from build123d import *

# Parameters (mm, degrees)
SKETCH2_R           = 1.55
CUT_EXTRUDE5_DEPTH  = 14.87
CUT_EXTRUDE10_DEPTH = 3.88
SKETCH5_R           = 3.26
CUT_EXTRUDE11_DEPTH = 2.18


with BuildPart() as part:
    # Sketch1 → Revolve1 (revolve)
    with BuildSketch(Plane.XY):
        with BuildLine():
            Line((0, 0.5), (5.525741394, 0.5))
            ThreePointArc((5.525741394, 0.5), (7.89, 0), (5.525741394, -0.5))
            Line((5.525741394, -0.5), (4.86, -0.5))
            ThreePointArc((4.86, -0.5), (4.294314575, -0.734314575), (4.06, -1.3))
            Line((4.06, -1.3), (4.06, -5.55))
            ThreePointArc((4.06, -5.55), (3.825685425, -6.115685425), (3.26, -6.35))
            Line((3.26, -6.35), (0, -6.35))
            Line((0, -6.35), (0, 0))
            Line((0, 0), (0, 0.5))
        make_face()
    revolve(axis=Axis((0, 0, 0), (0, 1, 0)))

    # Sketch2 → Cut-Extrude5 (cut)
    with BuildSketch(Plane(origin=(0, 0.5, 0), x_dir=(1, 0, 0), z_dir=(0, 1, 0))):
        with Locations(Location((0, 0, 0), (0, 0, 180))):
            Circle(SKETCH2_R)
    extrude(amount=-CUT_EXTRUDE5_DEPTH, mode=Mode.SUBTRACT)

    # Sketch3 → Cut-Extrude10 (cut)
    with BuildSketch(Plane(origin=(0, 0.5, 0), x_dir=(1, 0, 0), z_dir=(0, 1, 0))):
        with BuildLine():
            ThreePointArc((-2.210699096, 0.32868603), (-1.935566777, 1.1175), (-1.39, 1.750178562))
            Line((-1.39, 1.750178562), (-1.39, 5.3480574))
            ThreePointArc((-1.39, 5.3480574), (-4.785432422, 2.762870697), (-5.326553569, -1.470253389))
            Line((-5.326553569, -1.470253389), (-2.210699096, 0.32868603))
        make_face()
        with BuildLine():
            Line((1.39, 5.3480574), (1.39, 1.750178562))
            ThreePointArc((1.39, 1.750178562), (1.935566777, 1.1175), (2.210699096, 0.32868603))
            Line((2.210699096, 0.32868603), (5.326553569, -1.470253389))
            ThreePointArc((5.326553569, -1.470253389), (5.475718012, -0.741842439), (5.525741394, 0))
            ThreePointArc((5.525741394, 0), (4.371189683, 3.380313404), (1.39, 5.3480574))
        make_face()
        with BuildLine():
            ThreePointArc((0.820699096, -2.078864592), (0, -2.235), (-0.820699096, -2.078864592))
            Line((-0.820699096, -2.078864592), (-3.936553569, -3.877804011))
            ThreePointArc((-3.936553569, -3.877804011), (0, -5.525741394), (3.936553569, -3.877804011))
            Line((3.936553569, -3.877804011), (0.820699096, -2.078864592))
        make_face()
    extrude(amount=-CUT_EXTRUDE10_DEPTH, mode=Mode.SUBTRACT)

    # Sketch5 → Cut-Extrude11 (cut)
    with BuildSketch(Plane.XZ.offset(6.35)):
        Circle(SKETCH5_R)
    extrude(amount=-CUT_EXTRUDE11_DEPTH, mode=Mode.SUBTRACT)


solid = part.part
Design review of the part built by this model. Coordinates are the model's own, in mm. A direction names the side the tool comes from. Coordinates: 2 decimals unless noted, no trailing zeros. Order: outer loops, then holes, each group sorted by start corner. A loop starts at its lowest first (then second) coordinate and runs counter-clockwise, first axis right, second up. Notation, with made-up numbers: (-0.5, 39.25) - (14.5, 39.25) arc R12 ccw to (14.5, 46.25) - close; hole circle Ø11 at (-7.5, 59.5). An arc over 180 degrees is marked (long way). Put each result on its own line as item: value.
1) Tool access review of faces 4 (the face through (-4.5, -0.5, 2.6)), 5 (the face through (-1.39, -1, -3)), 6 (the face through (3, -3.38, -2)): name each direction out of +Z, -Z, +X, -X, +Y, -Y from which nothing blocks a thin tool from reaching the whole face with its end or side.
Response values:
face 4: -Y
face 5: +Y
face 6: -Z, +X, +Y
2) Wall thickness on L1, parallel to X at y = -5.5, z = 0; L2, parallel to Z at x = 0, y = -1.9 (3 decimals): over which ranges is each line inside the solid? List them lowest first. Write a range as from..to.
Response values:
L1: x = -4.06..-3.26, 3.26..4.06
L2: z = -4.06..-1.55, 1.55..2.235
3) Take a section at A-A, the plane x = 0. Give the boundary of the cut face in (y, z) (3 decimals).
Response values:
outline: (-6.35, -3.26) arc R0.8 ccw to (-5.55, -4.06) - (-1.3, -4.06) arc R0.8 cw to (-0.5, -4.86) - (-0.5, -5.526) arc R1.235 ccw (long way) to (0.5, -5.526) - (0.5, -1.55) - (-4.17, -1.55) - (-4.17, -3.26) - close; (-6.35, 3.26) - (-4.17, 3.26) - (-4.17, 1.55) - (0.5, 1.55) - (0.5, 2.235) - (-3.38, 2.235) - (-3.38, 4.06) - (-5.55, 4.06) arc R0.8 ccw to start; (-0.5, 5.526) - (0.5, 5.526) arc R1.235 ccw (long way) to start
4) Take a section at D-D, the plane z = -2. Count the separate pieces of the cut face and the enclosed holes in it, and give its area (3 significant figures).
Response values:
separate pieces: 3
enclosed holes: 0
area: 30.1 mm²
5) Take a section at C-C, the plane y = -2.25. Give the boundary of the cut face in (x, z) (3 decimals).
Response values:
outline: (-3.999, 0.704) - (-2.211, -0.329) arc R2.235 ccw to (-1.39, -1.75) - (-1.39, -3.815) arc R4.06 ccw to (1.39, -3.815) - (1.39, -1.75) arc R2.235 ccw to (2.211, -0.329) - (3.999, 0.704) arc R4.06 ccw to (2.609, 3.111) - (0.821, 2.079) arc R2.235 ccw to (-0.821, 2.079) - (-2.609, 3.111) arc R4.06 ccw to start; hole circle Ø3.1 at (0, 0)
6) Take a section at B-B, the plane y = -0.75. Give the boundary of the cut face in (x, z) (3 decimals), and give its area (3 significant figures).
Response values:
outline: circle Ø15.272 at (0, 0); (-4.2, 0.82) - (-2.211, -0.329) arc R2.235 ccw to (-1.39, -1.75) - (-1.39, -4.047) arc R4.279 ccw to (1.39, -4.047) - (1.39, -1.75) arc R2.235 ccw to (2.211, -0.329) - (4.2, 0.82) arc R4.279 ccw to (2.81, 3.227) - (0.821, 2.079) arc R2.235 ccw to (-0.821, 2.079) - (-2.81, 3.227) arc R4.279 ccw to start; hole circle Ø11.348 at (0, 0); hole circle Ø3.1 at (0, 0)
area: 108 mm²
7) The part is to be moulded in two halves that separate along Z. For faces 1 (the face through (3.873, -3.927, -1.22)), 2 (the face through (0, -3.38, 3)), 3 (the face through (4.4, -0.5, 2.5)), say which applies: released by +Z, released by -Z, zero draft, split by the parting line, or undercut.
Response values:
face 1: split by the parting line
face 2: zero draft
face 3: undercut
8) Insertion check: P1, Ø3, axis at x = 3, z = -2.5, coming from the +Y side; P2, Ø7.5, axis at x = 0, z = 0, coming from the -Y side; P3, Ø2, axis at x = -4, z = 2.5, coming from the -Y side; P4, Ø1, axis at x = -6, z = 5, coming from the +Y side. Each pin has a flat end and moves straight along its axis. Give the tip position at first contact, or say it passes through.
Response values:
P1: stops at y = -3.38
P2: stops at y = -6.35
P3: stops at y = -6.21
P4: stops at y = 1.05
